from build123d import *

# Parameters (mm, degrees)
F0_W     = 40
F0_H     = 25.95
F1_DEPTH = 5.3
F2_W     = 23
F2_H     = 25.95
F3_DEPTH = 2
F4_R     = 1.5


with BuildPart() as f1:
    # F0 (on Top) → F1 (new body)
    with BuildSketch(Plane.XY):
        with Locations((-40.170929, 36.161726)):
            Rectangle(F0_W, F0_H)
    extrude(amount=F1_DEPTH)

    # F2 (on face) → F3 (join)
    with BuildSketch(Plane.XY.offset(5.3)):
        with Locations((-31.670929, 36.161726)):
            Rectangle(F2_W, F2_H)
    extrude(amount=F3_DEPTH)

    # F4
    f4_edges = [f1.edges().sort_by_distance(p)[0] for p in [
        (-20.170929, 23.186726, 3.65),
        (-20.170929, 49.136726, 3.65),
        (-60.170929, 23.186726, 2.65),
        (-60.170929, 49.136726, 2.65),
    ]]
    fillet(f4_edges, radius=F4_R)


solid = f1.part
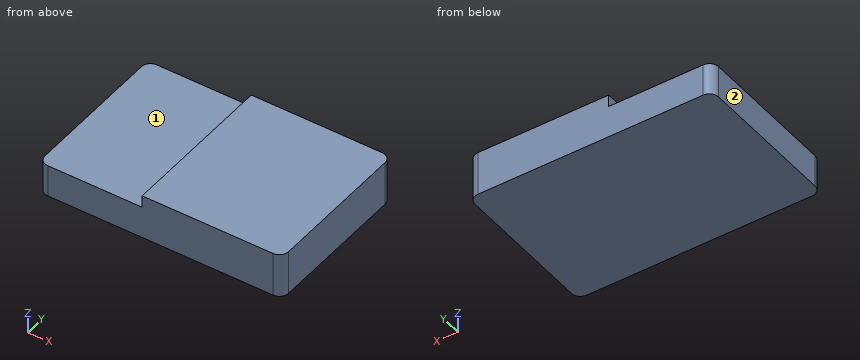
Work out the finished part from the listing and answer in its coordinate system (mm). Face numbers are marked on the shaded views. A direction names the side the tool comes from. Round coordinates to 2 decimals unless told otherwise and drop trailing zeros. Write each loop counter-clockwise with the first axis right and the second up, starting at its lowest first coordinate (ties: lowest second). Pieces come first, ordered by that corner, then holes.
1) Given pin 1 Ø3 at (x, y) = (-48, 37) entering from +Z; pin 2 Ø1.6 at (y, z) = (36.5, 6.5) entering from -X, each flat-ended and moving along its own axis, determine where each tip first touches the part or whether it passes through.
2) A cutting plane is placed at A-A (y = 46.5). Give the vertices of the cut face in (x, z), plus the area to 3 significant figures.
3) A tool of negligible diameter and unlimited length cuts with its end or side. For the marked faces 1 and 2, from which of +Z, -Z, +X, -X, +Y, -Y can it reach the whole face along a straight path? Write none if from no direction.
4) A cutting plane is placed at B-B (z = 6.25). Give the vertices of the cut face in (x, y), plus the area to 3 significant figures.
5) Straight lines are drawn through the part: line 1 (X direction, y = 29, z = 5.75); line 2 (Z direction, x = -53.5, y = 38). For each, find the intervals that lie inside material, in ascending order.
Completed:
1. pin 1: stops at z = 5.3
1. pin 2: stops at x = -43.17
2. outline: (-60.17, 0) - (-20.17, 0) - (-20.17, 7.3) - (-43.17, 7.3) - (-43.17, 5.3) - (-60.17, 5.3) - close
2. area: 258 mm2
3. face 1: +Z, -X, +Y, -Y
3. face 2: +Z, -Z, -X, +Y, -Y
4. outline: (-43.17, 23.19) - (-21.67, 23.19) arc R1.5 ccw to (-20.17, 24.69) - (-20.17, 47.64) arc R1.5 ccw to (-21.67, 49.14) - (-43.17, 49.14) - close
4. area: 596 mm2
5. line 1: x = -43.17 to -20.17
5. line 2: z = 0 to 5.3
